Read the model definition and answer for the solid it produces. Units are mm, in the model's axes. A direction names the side the tool comes from. Coordinates: 2 decimals unless noted, no trailing zeros. Loops run counter-clockwise (first coordinate to the right, second up) from the corner with the lowest first, then second, coordinate; pieces in that order, holes last. Notation, with made-up numbers: (32.25, 64) - (42.25, 64) arc R22 cw to (42.25, 87) - close; hole circle Ø9 at (80.5, -13). An arc over 180 degrees is marked (long way). One line per question, with ' | ' between items. Start each with the question number.
Autodesk Inventor part; units mm, degrees
ref_plane "Work Plane1" through (-24.9, -24.9, 7.7) normal (0, 0, 1) x (1, 0, 0)
ref_plane "YZ Plane" through (0, 0, 0) normal (1, 0, 0) x (0, 1, 0)
ref_plane "XZ Plane" through (0, 0, 0) normal (0, 1, 0) x (-1, 0, 0)
sketch "Sketch1" plane through (0, 0, 0) normal (0, 0, 1) x (1, 0, 0)
  circle A0 centre (-10, 20.9) radius 1.875
  circle A1 centre (-10, -20.9) radius 1.875
  circle A2 centre (10, 20.9) radius 1.875
  circle A3 centre (10, -20.9) radius 1.875
  circle A4 centre (20.8, -14.4) radius 2.075
  circle A5 centre (20.8, 14.4) radius 2.075
  circle A6 centre (-20.8, 14.4) radius 2.075
  circle A7 centre (-20.8, -14.4) radius 2.075
  line L0 (16.9, -16.9) -> (-16.9, -16.9)
  line L1 (-16.9, -16.9) -> (-16.9, 16.9)
  line L2 (-16.9, 16.9) -> (16.9, 16.9)
  line L3 (16.9, 16.9) -> (16.9, -16.9)
  line L4 (-17.05, 24.9) -> (-17.05, 22.55)
  line L5 (-17.05, 22.55) -> (-22.55, 17.05)
  line L6 (-22.55, 17.05) -> (-24.9, 17.05)
  line L7 (-24.9, 17.05) -> (-24.9, -17.05)
  line L8 (-24.9, -17.05) -> (-22.55, -17.05)
  line L9 (-22.55, -17.05) -> (-17.05, -22.55)
  line L10 (-17.05, -22.55) -> (-17.05, -24.9)
  line L11 (-17.05, -24.9) -> (17.05, -24.9)
  line L12 (17.05, -24.9) -> (17.05, -22.55)
  line L13 (17.05, -22.55) -> (22.55, -17.05)
  line L14 (22.55, -17.05) -> (24.9, -17.05)
  line L15 (24.9, -17.05) -> (24.9, 17.05)
  line L16 (24.9, 17.05) -> (22.55, 17.05)
  line L17 (22.55, 17.05) -> (17.05, 22.55)
  line L18 (17.05, 22.55) -> (17.05, 24.9)
  line L19 (17.05, 24.9) -> (-17.05, 24.9)
  line L20 (24.825, 16.975) -> (24.825, -16.975)
  line L21 (24.825, -16.975) -> (22.5189, -16.975)
  line L22 (22.5189, -16.975) -> (16.975, -22.5189)
  line L23 (16.975, -22.5189) -> (16.975, -24.825)
  line L24 (16.975, -24.825) -> (-16.975, -24.825)
  line L25 (-16.975, -24.825) -> (-16.975, -22.5189)
  line L26 (-16.975, -22.5189) -> (-22.5189, -16.975)
  line L27 (-22.5189, -16.975) -> (-24.825, -16.975)
  line L28 (-24.825, -16.975) -> (-24.825, 16.975)
  line L29 (-24.825, 16.975) -> (-22.5189, 16.975)
  line L30 (-22.5189, 16.975) -> (-16.975, 22.5189)
  line L31 (-16.975, 22.5189) -> (-16.975, 24.825)
  line L32 (-16.975, 24.825) -> (16.975, 24.825)
  line L33 (16.975, 24.825) -> (16.975, 22.5189)
  line L34 (16.975, 22.5189) -> (22.5189, 16.975)
  line L35 (22.5189, 16.975) -> (24.825, 16.975)
  point P0 (0, 0)
  dimension "d0" = 0.075
ref_plane "Work Plane1" through (-24.9, -24.9, 7.7) normal (0, 0, 1) x (1, 0, 0)
extrude "Extrusion1" add sketch "Sketch1" along normal blind 2.5 from surface at 7.7 contours A0 | A1 | A2 | A3 | A4 | A5 | A6 | A7 | L0 L1 L2 L3 | L20 L21 L22 L23 L24 L25 L26 L27 L28 L29 L30 L31 L32 L33 L34 L35
sketch "Sketch2" plane through (0, 0, 0) normal (0, 0, 1) x (1, 0, 0)
  line L0 (22.5189, 16.975) -> (24.825, 16.975)
  line L1 (16.975, 22.5189) -> (22.5189, 16.975)
  line L2 (16.975, 24.825) -> (16.975, 22.5189)
  line L3 (-16.975, 24.825) -> (16.975, 24.825)
  line L4 (-16.975, 22.5189) -> (-16.975, 24.825)
  line L5 (-22.5189, 16.975) -> (-16.975, 22.5189)
  line L6 (-24.825, 16.975) -> (-22.5189, 16.975)
  line L7 (-24.825, -16.975) -> (-24.825, 16.975)
  line L8 (-22.5189, -16.975) -> (-24.825, -16.975)
  line L9 (-16.975, -22.5189) -> (-22.5189, -16.975)
  line L10 (-16.975, -24.825) -> (-16.975, -22.5189)
  line L11 (16.975, -24.825) -> (-16.975, -24.825)
  line L12 (16.975, -22.5189) -> (16.975, -24.825)
  line L13 (22.5189, -16.975) -> (16.975, -22.5189)
  line L14 (24.825, -16.975) -> (22.5189, -16.975)
  line L15 (24.825, 16.975) -> (24.825, -16.975)
  line L16 (24.825, -16.975) -> (22.5189, -16.975)
  line L17 (22.5189, -16.975) -> (22.5189, 16.975)
  line L18 (22.5189, 16.975) -> (24.825, 16.975)
  line L19 (24.825, 16.975) -> (24.825, -16.975)
  line L20 (-22.5189, 16.975) -> (-24.825, 16.975)
  line L21 (-24.825, 16.975) -> (-24.825, -16.975)
  line L22 (-24.825, -16.975) -> (-22.5189, -16.975)
  line L23 (-22.5189, -16.975) -> (-22.5189, 16.975)
  line L24 (22.525, -14.675) -> (21.5662, -14.675)
  line L25 (21.5662, -14.675) -> (14.675, -21.5662)
  line L26 (14.675, -21.5662) -> (14.675, -22.525)
  line L27 (14.675, -22.525) -> (-14.675, -22.525)
  line L28 (-14.675, -22.525) -> (-14.675, -21.5662)
  line L29 (-14.675, -21.5662) -> (-21.5662, -14.675)
  line L30 (-21.5662, -14.675) -> (-22.525, -14.675)
  line L31 (-22.525, -14.675) -> (-22.525, 14.675)
  line L32 (-22.525, 14.675) -> (-21.5662, 14.675)
  line L33 (-21.5662, 14.675) -> (-14.675, 21.5662)
  line L34 (-14.675, 21.5662) -> (-14.675, 22.525)
  line L35 (-14.675, 22.525) -> (14.675, 22.525)
  line L36 (14.675, 22.525) -> (14.675, 21.5662)
  line L37 (14.675, 21.5662) -> (21.5662, 14.675)
  line L38 (21.5662, 14.675) -> (22.525, 14.675)
  line L39 (22.525, 14.675) -> (22.525, -14.675)
  line L40 (14.675, 22.525) -> (14.675, 24.825)
  line L41 (-14.675, 22.525) -> (-14.675, 24.825)
  line L42 (-14.675, -22.525) -> (-14.675, -24.825)
  line L43 (14.675, -22.525) -> (14.675, -24.825)
  point P0 (0, 0)
  dimension "d3" = 2.3
extrude "Extrusion2" add sketch "Sketch2" along normal blind 31.825 from surface at 10.2 contours L17 L38 L37 L36 L40 L3 L2 L1 | L0 L15 L14 L17 L24 L39 L38 | L17 L13 L12 L11 L43 L26 L25 L24 | L41 L34 L33 L32 L23 L5 L4 L3 | L42 L11 L10 L9 L23 L30 L29 L28 | L23 L32 L31 L30 L8 L7 L6
extrude "Extrusion3" add sketch "Sketch2" against normal blind 2.5 from surface at 42.025
properties part number "Tunnel Horizontal"
1) Given pin 1 Ø0.7 at (y, z) = (24, 28.5) entering from -X (3 decimals); pin 2 Ø1.8 at (x, z) = (-24, 29) entering from -Y (3 decimals); pin 3 Ø1 at (y, z) = (-23.5, 23) entering from +X (3 decimals), each flat-ended and moving along its own axis, determine where each tip first touches the part or whether it passes through.
2) The part is cut by section C-C on y = 12.5. Write down the section's boundary in (x, z) (3 decimals), and give its area (3 significant figures).
3) The part is cut by section B-B on x = 5. Write down the section's boundary in (y, z) (3 decimals), and give its area (3 significant figures).
4) Which of the six approach directions +Z, -Z, +X, -X, +Y, -Y give full straight-line access (tool end or side, diameter ignored) to faces 4 (the flat face through (-16.975, 24, 25)), 5 (the flat face through (-16.975, -24, 25)), 6 (the flat face through (14.675, -23, 25)), 7 (the flat face through (-18.07, -18.17, 24.66))?
5) The mould has two halves that part along Y. Classify faces 1 (the flat face through (-19.708, -19.786, 24.622)), 2 (the flat face through (0, 0, 7.7)), 3 (the flat face through (-18.17, 18.07, 24.66)): released by +Y, released by -Y, zero draft, split by the parting line, or undercut.
6) Find the intervals of material crossed by line 1 along Z through (x, y) = (19, 5) (3 decimals); line 2 along X through (y, z) = (4, 22) (3 decimals); line 3 along Y through (x, z) = (17.5, 31.5), in increasing order. Write a range as from..to.
7) The part is cut by section D-D on x = 20. Write down the section's boundary in (y, z) (3 decimals), and give its area (3 significant figures).
Answer below:
1) pin 1: x = -16.975 | pin 2: y = -16.975 | pin 3: x = 16.975
2) outline: (-24.825, 7.7) - (24.825, 7.7) - (24.825, 42.025) - (-24.825, 42.025) - close; hole (-22.525, 10.2) - (22.525, 10.2) - (22.525, 39.525) - (-22.525, 39.525) - close | area: 383 mm2
3) outline: (-24.825, 7.7) - (24.825, 7.7) - (24.825, 10.2) - (-24.825, 10.2) - close; (-24.825, 39.525) - (24.825, 39.525) - (24.825, 42.025) - (-24.825, 42.025) - close | area: 248 mm2
4) face 4: +Z, -Z, -X, +Y | face 5: +Z, -Z, -X, -Y | face 6: +Y, -Y | face 7: none
5) face 1: released by -Y | face 2: zero draft | face 3: undercut
6) line 1: 7.7..10.2, 39.525..42.025 | line 2: -24.825..-22.525, 22.525..24.825 | line 3: -21.99..-18.74, 18.74..21.99
7) outline: (-19.494, 7.7) - (19.494, 7.7) - (19.494, 42.025) - (-19.494, 42.025) - close; hole (-16.241, 10.2) - (16.241, 10.2) - (16.241, 39.525) - (-16.241, 39.525) - close | area: 386 mm2
